```python
from build123d import *

# Parameters (mm, degrees)
F0_R     = 7.5
F0_R_2   = 5.5
F0_R_3   = 4.5
F1_DEPTH = 1
F3_DEPTH = 12
F4_DEPTH = 19.5


with BuildPart() as f1:
    # F0 (on Top) → F1 (new body)
    with BuildSketch(Plane.XY):
        Circle(F0_R)
        Circle(F0_R_2, mode=Mode.SUBTRACT)
        Circle(F0_R_2)
        Circle(F0_R_3, mode=Mode.SUBTRACT)
        Circle(F0_R_3)
        with BuildLine():
            ThreePointArc((-2.284732, -2.45), (-3.35, 0), (-2.284732, 2.45))
            Line((-2.284732, 2.45), (2.284732, 2.45))
            ThreePointArc((2.284732, 2.45), (3.35, 0), (2.284732, -2.45))
            Line((2.284732, -2.45), (-2.284732, -2.45))
        make_face(mode=Mode.SUBTRACT)
    extrude(amount=F1_DEPTH)



with BuildPart() as f2_1:
    # F2: copy of F1
    add(f1.part.moved(Location((0, 0, 10))))


with BuildPart() as f3:
    # F0 (on Top) → F3 (new body)
    with BuildSketch(Plane.XY):
        Circle(F0_R_2)
        Circle(F0_R_3, mode=Mode.SUBTRACT)
        Circle(F0_R_3)
        with BuildLine():
            ThreePointArc((-2.284732, -2.45), (-3.35, 0), (-2.284732, 2.45))
            Line((-2.284732, 2.45), (2.284732, 2.45))
            ThreePointArc((2.284732, 2.45), (3.35, 0), (2.284732, -2.45))
            Line((2.284732, -2.45), (-2.284732, -2.45))
        make_face(mode=Mode.SUBTRACT)
    extrude(amount=F3_DEPTH)


with BuildPart() as f1_1:
    add(f1.part)

    add(f2_1.part)  # F4 merges F2_1

    add(f3.part)  # F4 merges F3
    # F0 (on Top) → F4 (join)
    with BuildSketch(Plane.XY):
        Circle(F0_R_3)
        with BuildLine():
            ThreePointArc((-2.284732, -2.45), (-3.35, 0), (-2.284732, 2.45))
            Line((-2.284732, 2.45), (2.284732, 2.45))
            ThreePointArc((2.284732, 2.45), (3.35, 0), (2.284732, -2.45))
            Line((2.284732, -2.45), (-2.284732, -2.45))
        make_face(mode=Mode.SUBTRACT)
    extrude(amount=F4_DEPTH)

    # F5 (on Front) → F6 (revolve)
    with BuildSketch(Plane.XZ):
        Polygon((4.75, 18.75), (4.5, 19.5), (4.5, 18), align=None)
    revolve(axis=Axis((0, 0, 8.754228), (0, 0, 1)))


solid = f1_1.part
```
Here's how the part is built. I have some questions about the finished solid (model axes, mm). A direction names the side the tool comes from. Give positions to 0.01 mm unless a question says otherwise; leave off trailing zeros. Loops run counter-clockwise (first coordinate to the right, second up) from the corner with the lowest first, then second, coordinate; pieces in that order, holes last. Notation, with made-up numbers: (-29.5, 15) -> (-14.5, 15) arc R34 cw to (-14.5, 45) -> close; hole circle Ø1 at (59, 51). An arc over 180 degrees is marked (long way). Use one line per item in the form item = value. Start each with the question number.
1) Imagine slicing it at C-C (z = 6.5). Please give me the cut outline in (x, y).
2) Imagine slicing it at B-B (x = 0). Please give me the cut outline in (y, z).
3) For P1, Ø1.4, axis at x = -0.5, z = 7, coming from the +Y side; P2, Ø4, axis at y = -4, z = 12.5, coming from the -X side; P3, Ø6, axis at y = 0.5, z = 17.5, coming from the -X side, each with a flat end and sliding along its axis, tell me the tip position at first contact or that it passes through.
4) Please list where these lines run through material, in increasing order: line 1 along Z through (x, y) = (3.5, -4.5); line 2 along Y through (x, z) = (-0.25, 8.5); line 3 along Y through (x, z) = (-1, 16.75).
5) Thinking about a two-plate mould opening in X: for faces 1 (the face through (3.35, 0.04, 9.61)), 2 (the face through (-5, 0, 12)), 3 (the face through (-1.19, -5.37, 11.49)), which applies, +X half, -X half, draft (parallel to the pull), parting line (faces both ways), or undercut?
6) Imagine slicing it at D-D (y = 6.75). Please give me the cut outline in (x, z).
7) Imagine slicing it at A-A (y = 0). Please give me the cut outline in (x, z), then the cut area to 3 significant figures.
8) Which directions (+Z, -Z, +X, -X, +Y, -Y) give clear straight access to the entire face, cutting with the end or side of a thin tool? Please do faces 4 (the face through (-4, 4, 1)), 5 (the face through (-4, 4, 11)), 6 (the face through (0, 2.45, 10)).
Check values:
q1.outline = circle Ø11 at (0, 0); hole (-2.28, -2.45) -> (2.28, -2.45) arc R3.35 ccw to (2.28, 2.45) -> (-2.28, 2.45) arc R3.35 ccw to start
q2.outline = (-7.5, 0) -> (-2.45, 0) -> (-2.45, 19.5) -> (-4.5, 19.5) -> (-4.75, 18.75) -> (-4.5, 18) -> (-4.5, 12) -> (-5.5, 12) -> (-5.5, 11) -> (-7.5, 11) -> (-7.5, 10) -> (-5.5, 10) -> (-5.5, 1) -> (-7.5, 1) -> close; (2.45, 0) -> (7.5, 0) -> (7.5, 1) -> (5.5, 1) -> (5.5, 10) -> (7.5, 10) -> (7.5, 11) -> (5.5, 11) -> (5.5, 12) -> (4.5, 12) -> (4.5, 18) -> (4.75, 18.75) -> (4.5, 19.5) -> (2.45, 19.5) -> close
q3.P1 = 5.5
q3.P2 = -7.01
q3.P3 = -4.75
q4.line_1 = 0 to 1, 10 to 11
q4.line_2 = -5.49 to -2.45, 2.45 to 5.49
q4.line_3 = -4.39 to -2.45, 2.45 to 4.39
q5.face_1 = undercut
q5.face_2 = draft
q5.face_3 = parting line
q6.outline = (-3.27, 0) -> (3.27, 0) -> (3.27, 1) -> (-3.27, 1) -> close; (-3.27, 10) -> (3.27, 10) -> (3.27, 11) -> (-3.27, 11) -> close
q7.outline = (-7.5, 0) -> (-3.35, 0) -> (-3.35, 19.5) -> (-4.5, 19.5) -> (-4.75, 18.75) -> (-4.5, 18) -> (-4.5, 12) -> (-5.5, 12) -> (-5.5, 11) -> (-7.5, 11) -> (-7.5, 10) -> (-5.5, 10) -> (-5.5, 1) -> (-7.5, 1) -> close; (3.35, 0) -> (7.5, 0) -> (7.5, 1) -> (5.5, 1) -> (5.5, 10) -> (7.5, 10) -> (7.5, 11) -> (5.5, 11) -> (5.5, 12) -> (4.5, 12) -> (4.5, 18) -> (4.75, 18.75) -> (4.5, 19.5) -> (3.35, 19.5) -> close
q7.area = 77.2 mm^2
q8.face_4 = none
q8.face_5 = +Z
q8.face_6 = +Z, -Z
